from build123d import *

# Parameters (mm, degrees)
SKETCH1_W           = 200
SKETCH1_H           = 85
BOSS_EXTRUDE1_DEPTH = 10
SKETCH2_R           = 7.5
CUT_EXTRUDE1_DEPTH  = 10


with BuildPart() as part:
    # Sketch1 → Boss-Extrude1 (new body)
    with BuildSketch(Plane(origin=(0, 0, 0), x_dir=(1, 0, 0), z_dir=(0, 1, 0))):
        Rectangle(SKETCH1_W, SKETCH1_H)
    extrude(amount=BOSS_EXTRUDE1_DEPTH)

    # Sketch2 → Cut-Extrude1 (cut)
    with BuildSketch(Plane(origin=(0, 10, 0), x_dir=(1, 0, 0), z_dir=(0, 1, 0))):
        with Locations(Location((-60, 21.5, 0), (0, 0, 270))):
            Circle(SKETCH2_R)
    cut_extrude1 = extrude(amount=-CUT_EXTRUDE1_DEPTH, mode=Mode.SUBTRACT)

    # Mirror1: Cut-Extrude1 across plane
    add(cut_extrude1.mirror(Plane(origin=(0, 0, 0), x_dir=(0, 0, 1), z_dir=(1, 0, 0))), mode=Mode.SUBTRACT)


solid = part.part
Source: CAD feature listing. Evaluate the final solid. Frame: model axes, mm. Give positions to 0.01 mm unless a question says otherwise; leave off trailing zeros. Write each loop counter-clockwise with the first axis right and the second up, starting at its lowest first coordinate (ties: lowest second). Pieces come first, ordered by that corner, then holes. Notation, with made-up numbers: (75.5, 78.25) - (90.5, 78.25) arc R13 ccw to (90.5, 86.25) - close; hole circle Ø6 at (19, -7.75). An arc over 180 degrees is marked (long way). Write item = value, one per line. Start each with the question number.
Q1. Draft query along Z for faces 1 (the flat face through (100, 5, 1)), 2 (the cylindrical face through (54.9, 5.1, -27)), 3 (the flat face through (-1, 5, -42.5)). Return one class per face: +Z half, -Z half, draft (parallel to the pull), parting line (faces both ways), or undercut.
Q2. Cut plane C-C, the plane y = 7. Return loops of the section in (x, z), then the cut area to 3 significant figures.
Q3. Pin query (flat end, axial travel): pin 1 Ø13.5 at (x, z) = (-60, -21.5) entering from +Y. Return the tip coordinate at first contact, or that it passes through.
Q4. Cut plane B-B, the plane x = -60. Return loops of the section in (y, z).
Q5. Cut plane A-A, the plane z = -21.5. Return loops of the section in (x, y).
Q6. Material intervals for probe 1 along X at (y, z) = (7, -21.5); probe 2 along Z at (x, y) = (60.5, 2), sorted ascending.
Computed values:
q1.face_1 = draft
q1.face_2 = undercut
q1.face_3 = -Z half
q2.outline = (-100, -42.5) - (100, -42.5) - (100, 42.5) - (-100, 42.5) - close; hole circle Ø15 at (-60, -21.5); hole circle Ø15 at (60, -21.5)
q2.area = 16,600 mm²
q3.pin_1 = through
q4.outline = (0, -42.5) - (10, -42.5) - (10, -29) - (0, -29) - close; (0, -14) - (10, -14) - (10, 42.5) - (0, 42.5) - close
q5.outline = (-100, 0) - (-67.5, 0) - (-67.5, 10) - (-100, 10) - close; (-52.5, 0) - (52.5, 0) - (52.5, 10) - (-52.5, 10) - close; (67.5, 0) - (100, 0) - (100, 10) - (67.5, 10) - close
q6.probe_1 = -100 to -67.5, -52.5 to 52.5, 67.5 to 100
q6.probe_2 = -42.5 to -28.98, -14.02 to 42.5
